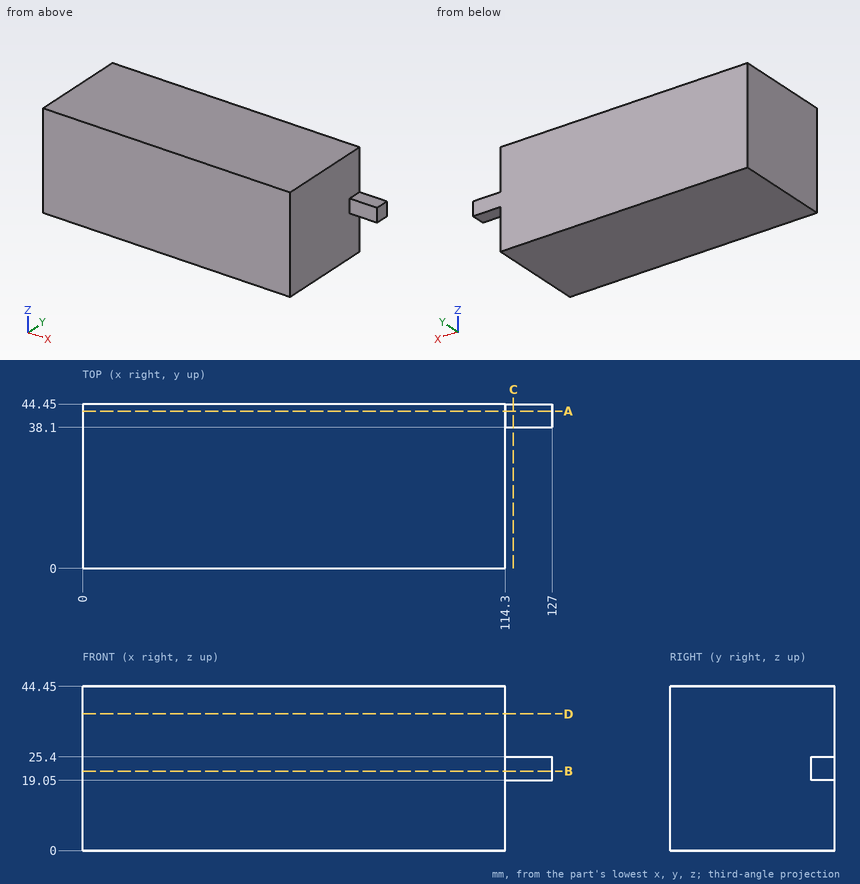
Check sheet for the drawn part. Datum: minimum x, y, z corner. Units: mm. Give positions to 0.01 mm unless a question says otherwise; leave off trailing zeros. Order: outer loops, then holes, each group sorted by start corner. A loop starts at its lowest first (then second) coordinate and runs counter-clockwise, first axis right, second up.
1. Sectioned sample at A-A (y = 42.5). Record the boundary of the cut face in (x, z).
Completed:
outline: (0, 0) - (114.3, 0) - (114.3, 19.05) - (127, 19.05) - (127, 25.4) - (114.3, 25.4) - (114.3, 44.45) - (0, 44.45) - close
2. Sectioned sample at B-B (z = 21.5). Record the boundary of the cut face in (x, y).
Completed:
outline: (0, 0) - (114.3, 0) - (114.3, 38.1) - (127, 38.1) - (127, 44.45) - (0, 44.45) - close
3. Sectioned sample at C-C (x = 116.5). Record the boundary of the cut face in (y, z).
Completed:
outline: (38.1, 19.05) - (44.45, 19.05) - (44.45, 25.4) - (38.1, 25.4) - close
4. Sectioned sample at D-D (z = 37). Record the boundary of the cut face in (x, y).
Completed:
outline: (0, 0) - (114.3, 0) - (114.3, 44.45) - (0, 44.45) - close
5. Scan lines: line 1 (X direction, y = 39.5, z = 2.5); line 2 (Z direction, x = 114.5, y = 39). Record each from-to range of solid material in increasing order.
Completed:
line 1: x = 0 to 114.3
line 2: z = 19.05 to 25.4
6. Depth check by flat-ended pin: pin 1 (1.9 mm diameter, centred on x = 122.5, y = 40, fed in from -Z); pin 2 (1 mm diameter, centred on x = 38.5, y = 33.5, fed in from -Z); pin 3 (12 mm diameter, centred on y = 23.5, z = 6.5, fed in from +X); pin 4 (3 mm diameter, centred on x = 123, z = 23, fed in from -Y). Enter the tip coordinate at first touch or a pass-through.
Completed:
pin 1: stops at z = 19.05
pin 2: stops at z = 0
pin 3: stops at x = 114.3
pin 4: stops at y = 38.1
